Verification items for the finished model (mm, model axes). A direction names the side the tool comes from. Round coordinates to 2 decimals unless told otherwise and drop trailing zeros. Loops run counter-clockwise (first coordinate to the right, second up) from the corner with the lowest first, then second, coordinate; pieces in that order, holes last. Notation, with made-up numbers: M 35,46 L 54,46 A16 ccw 54,75 Z; hole C 48.25,76.5 d6. An arc over 180 degrees is marked long. Answer as CSV lines item,"result".
```python
from build123d import *

# Parameters (mm, degrees)
F1_R     = 50.6050754874
F2_DEPTH = 6.35
F0_R     = 10.9982
F3_DEPTH = 6.35


with BuildPart() as f2:
    # F1 (on Front) → F2 (new body)
    with BuildSketch(Plane.XZ):
        Circle(F1_R)
        with BuildLine():
            add(Edge.make_bspline(
                [(-1.7389111535, -33.8362334716), (-3.1769237644, -33.1629443301), (-4.6149363754, -33.1629443301)],
                knots=[0, 0, 0, 1, 1, 1], degree=2))
            add(Edge.make_bspline(
                [(-4.6149363754, -33.1629443301), (-6.7013014931, -33.1629443301), (-7.9093429158, -34.5524690399)],
                knots=[0, 0, 0, 1, 1, 1], degree=2))
            add(Edge.make_bspline(
                [(-7.9093429158, -34.5524690399), (-9.1173843385, -35.9419937498), (-9.1173843385, -38.3580765952)],
                knots=[0, 0, 0, 1, 1, 1], degree=2))
            add(Edge.make_bspline(
                [(-9.1173843385, -38.3580765952), (-9.1173843385, -40.8406571336), (-7.9522893425, -42.196932997)],
                knots=[0, 0, 0, 1, 1, 1], degree=2))
            add(Edge.make_bspline(
                [(-7.9522893425, -42.196932997), (-6.7871943465, -43.5532088603), (-4.6315607987, -43.5532088603)],
                knots=[0, 0, 0, 1, 1, 1], degree=2))
            add(Edge.make_bspline(
                [(-4.6315607987, -43.5532088603), (-3.3071484132, -43.5532088603), (-1.6086865047, -43.0766420605)],
                knots=[0, 0, 0, 1, 1, 1], degree=2))
            Line((-1.6086865047, -43.0766420605), (-1.6086865047, -44.3650348623))
            add(Edge.make_bspline(
                [(-1.6086865047, -44.3650348623), (-2.9247866785, -44.8609968225), (-4.8559905125, -44.8609968225)],
                knots=[0, 0, 0, 1, 1, 1], degree=2))
            add(Edge.make_bspline(
                [(-4.8559905125, -44.8609968225), (-7.6516643555, -44.8609968225), (-9.1714137141, -43.162534914)],
                knots=[0, 0, 0, 1, 1, 1], degree=2))
            add(Edge.make_bspline(
                [(-9.1714137141, -43.162534914), (-10.6911630727, -41.4640730054), (-10.6911630727, -38.3386814348)],
                knots=[0, 0, 0, 1, 1, 1], degree=2))
            add(Edge.make_bspline(
                [(-10.6911630727, -38.3386814348), (-10.6911630727, -36.3825409659), (-9.9596884498, -34.9112795084)],
                knots=[0, 0, 0, 1, 1, 1], degree=2))
            add(Edge.make_bspline(
                [(-9.9596884498, -34.9112795084), (-9.2282138268, -33.4400180509), (-7.8470013286, -32.6434311036)],
                knots=[0, 0, 0, 1, 1, 1], degree=2))
            add(Edge.make_bspline(
                [(-7.8470013286, -32.6434311036), (-6.4657888304, -31.8468441563), (-4.595541215, -31.8468441563)],
                knots=[0, 0, 0, 1, 1, 1], degree=2))
            add(Edge.make_bspline(
                [(-4.595541215, -31.8468441563), (-2.6061518996, -31.8468441563), (-1.1154952816, -32.5727773048)],
                knots=[0, 0, 0, 1, 1, 1], degree=2))
            Line((-1.1154952816, -32.5727773048), (-1.7389111535, -33.8362334716))
        make_face(mode=Mode.SUBTRACT)
        with BuildLine():
            Line((5.2682832457, -39.4220396831), (2.6249999492, -39.4220396831))
            Line((2.6249999492, -39.4220396831), (2.6249999492, -44.6864403784))
            Line((2.6249999492, -44.6864403784), (1.1537384918, -44.6864403784))
            Line((1.1537384918, -44.6864403784), (1.1537384918, -32.0269420748))
            Line((1.1537384918, -32.0269420748), (4.6254722135, -32.0269420748))
            add(Edge.make_bspline(
                [(4.6254722135, -32.0269420748), (6.9556622055, -32.0269420748), (8.0681131945, -32.9191194558)],
                knots=[0, 0, 0, 1, 1, 1], degree=2))
            add(Edge.make_bspline(
                [(8.0681131945, -32.9191194558), (9.1805641835, -33.8112968368), (9.1805641835, -35.6039638104)],
                knots=[0, 0, 0, 1, 1, 1], degree=2))
            add(Edge.make_bspline(
                [(9.1805641835, -35.6039638104), (9.1805641835, -38.1142517209), (6.6342566893, -38.9981168903)],
                knots=[0, 0, 0, 1, 1, 1], degree=2))
            Line((6.6342566893, -38.9981168903), (10.0727415645, -44.6864403784))
            Line((10.0727415645, -44.6864403784), (8.3327185979, -44.6864403784))
            Line((8.3327185979, -44.6864403784), (5.2682832457, -39.4220396831))
        make_face(mode=Mode.SUBTRACT)
        Polygon((14.4366526672, -44.6864403784), (12.8434787726, -44.6864403784), (18.0884843075, -33.3513544602), (11.1893486594, -33.3513544602), (11.1893486594, -32.0269420748), (19.6123897719, -32.0269420748), (19.6123897719, -33.1795687533), align=None, mode=Mode.SUBTRACT)
    extrude(amount=F2_DEPTH)

    # F0 (on Front) → F3 (cut)
    with BuildSketch(Plane.XZ):
        with Locations((0, 31.75)):
            Circle(F0_R)
        Circle(F0_R)
        with Locations((-27.4963065702, -15.875)):
            Circle(F0_R)
        with Locations((27.4963065702, -15.875)):
            Circle(F0_R)
    extrude(amount=F3_DEPTH, mode=Mode.SUBTRACT)


solid = f2.part
```
1) Section check C-C (y = -1.25). State how many separate pieces and enclosed holes the cut face has, plus the area to 3 significant figures.
Here are the results:
separate pieces,"1"
enclosed holes,"7"
area,"6,390 mm^2"
2) Section check B-B (x = -18). Record the cut outline in (y, z), plus the area to 3 significant figures.
Here are the results:
outline,"M -6.35,-47.3 L 0,-47.3 L 0,-21.42 L -6.35,-21.42 Z; M -6.35,-10.33 L 0,-10.33 L 0,47.3 L -6.35,47.3 Z"
area,"530 mm^2"
3) Section check D-D (z = 15). Record the cut outline in (x, y).
Here are the results:
outline,"M -48.33,-6.35 L 48.33,-6.35 L 48.33,0 L -48.33,0 Z"
4) Material ranges on probe 1 along Z at (x, y) = (-6.5, -4.75); probe 2 along Z at (x, y) = (6, -1); probe 3 along X at (y, z) = (-6, 6), recorded low to high.
Here are the results:
probe 1,"z = -50.19 to -44.69, -43.23 to -33.52, -32.09 to -8.87, 8.87 to 22.88, 40.62 to 50.19"
probe 2,"z = -50.25 to -40.68, -32.12 to -9.22, 9.22 to 22.53, 40.97 to 50.25"
probe 3,"x = -50.25 to -9.22, 9.22 to 50.25"
5) Section check A-A (z = 0). Record the cut outline in (x, y).
Here are the results:
outline,"M -50.61,-6.35 L -11,-6.35 L -11,0 L -50.61,0 Z; M 11,-6.35 L 50.61,-6.35 L 50.61,0 L 11,0 Z"
6) Go/stop test with flat-tipped pins: pin 1 (1.9 mm diameter, centred on x = 16, y = -2, fed in from +Z); pin 2 (1.9 mm diameter, centred on y = -3, z = -40, fed in from +X); pin 3 (0.6 mm diameter, centred on y = -2, z = -43.5, fed in from -X). Record where each tip stops, or that it passes through.
Here are the results:
pin 1,"stops at z = 48.32"
pin 2,"stops at x = 32.19"
pin 3,"stops at x = -26.36"
7) Draft check along Z on faces 3 (the flat face through (-1, 0, 12)), 4 (the cylindrical face through (18.77, -3.13, -22.57)), 5 (the cylindrical face through (-37.3, -3.1, 34.2)). Enter one of: +Z half, -Z half, draft (parallel to the pull), parting line (faces both ways), or undercut.
Here are the results:
face 3,"draft"
face 4,"undercut"
face 5,"parting line"
8) Set-up check for faces 1 (the flat face through (-1, -6.35, 12)), 2 (the flat face through (15.43, -3.13, -39.1)): record each of +Z, -Z, +X, -X, +Y, -Y from which the full face is reachable in a straight line by a thin tool's end or side.
Here are the results:
face 1,"+Z, -Z, +X, -X, -Y"
face 2,"+Y, -Y"
